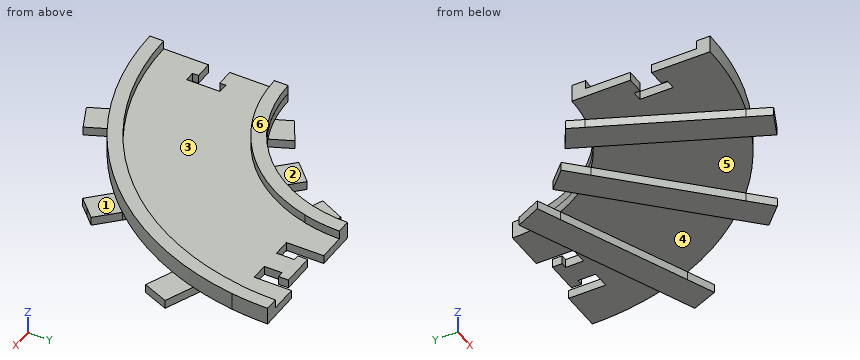
from build123d import *

# Parameters (mm, degrees)
F1_DEPTH  = 3.175
F2_W      = 14.0813224944
F2_H      = 13.6506203337
F3_DEPTH  = 3.175
F5_DEPTH  = 3.175
F2_W_2    = 4.1719265282
F6_DEPTH  = 25.4
F8_DEPTH  = 6.35
F9_DEPTH  = 3.175
F11_DEPTH = 25.4
F13_DEPTH = 3.175


with BuildPart() as f1:
    # F0 (on Top) → F1 (new body)
    with BuildSketch(Plane.XY):
        with BuildLine():
            Line((0, -51.2956328023), (0, -102.09075941))
            ThreePointArc((0, -102.09075941), (72.1890682753, -72.1890682753), (102.09075941, 0))
            Line((102.09075941, 0), (51.2956328023, 0))
            ThreePointArc((51.2956328023, 0), (36.2714897998, -36.2714897998), (0, -51.2956328023))
        make_face()
    extrude(amount=F1_DEPTH)

    # F2 (on Top) → F3 (join)
    with BuildSketch(Plane.XY):
        Polygon((70.5449951161, -7.1183972853), (72.7547951161, -7.1183972853), (72.7547951161, -13.6506203337), (80.5461628969, -13.6506203337), (80.5461628969, -7.1183972853), (82.7559628969, -7.1183972853), (82.7559628969, -3.5022496107), (70.5449951161, -3.5022496107), align=None)
        Polygon((51.7481602728, -13.6506203337), (66.4398123863, -13.6506203337), (66.3695515009, 0), (51.7481602728, 0), align=None)
        with Locations((93.9881238623, -6.8253101669)):
            Rectangle(F2_W, F2_H)
    extrude(amount=F3_DEPTH)

    # F4 (on face) → F5 (join)
    with BuildSketch(Plane.XY.offset(3.175)):
        with BuildLine():
            ThreePointArc((0, -56.3756328023), (39.8635922482, -39.8635922482), (56.3756328023, 0))
            Line((56.3756328023, 0), (51.3330261441, 0))
            ThreePointArc((51.3330261441, 0), (36.2979308853, -36.2979308853), (0, -51.3330261441))
            Line((0, -51.3330261441), (0, -56.3756328023))
        make_face()
        with BuildLine():
            Line((102.09075941, 0), (97.01075941, 0))
            ThreePointArc((97.01075941, 0), (68.5969658269, -68.5969658269), (0, -97.01075941))
            Line((0, -97.01075941), (0, -102.09075941))
            ThreePointArc((0, -102.09075941), (72.1890682753, -72.1890682753), (102.09075941, 0))
        make_face()
    extrude(amount=F5_DEPTH)

    # F2 (on Top) → F6 (cut)
    with BuildSketch(Plane.XY):
        Polygon((51.7481602728, -13.6506203337), (66.4398123863, -13.6506203337), (66.3695515009, 0), (51.7481602728, 0), align=None)
        Polygon((72.7547951161, -13.6506203337), (72.7547951161, -7.1183972853), (70.5449951161, -7.1183972853), (70.5449951161, -3.5022496107), (82.7559628969, -3.5022496107), (82.7559628969, -7.1183972853), (80.5461628969, -7.1183972853), (80.5461628969, -13.6506203337), (86.9474626151, -13.6506203337), (86.9474626151, 0), (76.6565515009, 0), (66.3695515009, 0), (66.4398123863, -13.6506203337), align=None)
        with Locations((93.9881238623, -6.8253101669)):
            Rectangle(F2_W, F2_H)
        with Locations((49.6621970087, -6.8253101669)):
            Rectangle(F2_W_2, F2_H)
    extrude(amount=F6_DEPTH, mode=Mode.SUBTRACT)

    # F7 (on Top) → F8 (join)
    with BuildSketch(Plane.XY):
        with BuildLine():
            ThreePointArc((54.7619331998, -13.660392724), (56.0189261095, -6.8815386855), (56.4400182242, 0))
            Line((56.4400182242, 0), (51.3051767249, 0))
            ThreePointArc((51.3051767249, 0), (50.8400637591, -6.8926827684), (49.4531579316, -13.660392724))
            Line((49.4531579316, -13.660392724), (54.7619331998, -13.660392724))
        make_face()
        with BuildLine():
            Line((102.1051767249, 0), (97.1390098326, 0))
            ThreePointArc((97.1390098326, 0), (96.8973822865, -6.8472284381), (96.1737017167, -13.660392724))
            Line((96.1737017167, -13.660392724), (101.1872560388, -13.660392724))
            ThreePointArc((101.1872560388, -13.660392724), (101.8754380952, -6.8455990928), (102.1051767249, 0))
        make_face()
    extrude(amount=F8_DEPTH)

    # F2 (on Top) → F9 (join)
    with BuildSketch(Plane.XY):
        with Locations((93.9881238623, -6.8253101669)):
            Rectangle(F2_W, F2_H)
        Polygon((51.7481602728, -13.6506203337), (66.4398123863, -13.6506203337), (66.3695515009, 0), (51.7481602728, 0), align=None)
    extrude(amount=F9_DEPTH)

    # F10 (on face) → F11 (cut)
    with BuildSketch(Plane.XY.offset(3.175)):
        Polygon((6.3110076786, -72.776100911), (0, -72.776100911), (0, -80.5674686917), (6.3110076786, -80.5674686917), (6.3110076786, -82.7772686917), (10.0084030033, -82.7772686917), (10.0084030033, -70.566300911), (6.3110076786, -70.566300911), align=None)
    extrude(amount=-F11_DEPTH, mode=Mode.SUBTRACT)

    # F12 (on face) → F13 (join)
    with BuildSketch(Plane(origin=(0, 0, 0), x_dir=(1, 0, 0), z_dir=(0, 0, -1))):
        with BuildLine():
            ThreePointArc((39.6434592285, 32.5520826521), (37.980845771, 34.4774897449), (36.2248193412, 36.3181002847))
            Line((36.2248193412, 36.3181002847), (29.0498583475, 29.1246633635))
            Line((29.0498583475, 29.1246633635), (32.646576808, 25.5371828667))
            Line((32.646576808, 25.5371828667), (39.6434592285, 32.5520826521))
        make_face()
        with BuildLine():
            Line((29.0498583475, 29.1246633635), (36.2248193412, 36.3181002847))
            ThreePointArc((36.2248193412, 36.3181002847), (34.3796988436, 38.0693873344), (32.4500223073, 39.7270436459))
            Line((32.4500223073, 39.7270436459), (25.4531398869, 32.7121438604))
            Line((25.4531398869, 32.7121438604), (29.0498583475, 29.1246633635))
        make_face()
        with BuildLine():
            Line((36.2248193412, 36.3181002847), (72.0961827352, 72.2818344532))
            ThreePointArc((72.0961827352, 72.2818344532), (70.2749350461, 74.0537417095), (68.4101530773, 75.7797737714))
            Line((68.4101530773, 75.7797737714), (32.4500223073, 39.7270436459))
            ThreePointArc((32.4500223073, 39.7270436459), (34.3796988436, 38.0693873344), (36.2248193412, 36.3181002847))
        make_face()
        with BuildLine():
            ThreePointArc((75.6035899985, 68.6048127777), (73.8727679087, 70.4651496728), (72.0961827352, 72.2818344532))
            Line((72.0961827352, 72.2818344532), (36.2248193412, 36.3181002847))
            ThreePointArc((36.2248193412, 36.3181002847), (37.980845771, 34.4774897449), (39.6434592285, 32.5520826521))
            Line((39.6434592285, 32.5520826521), (75.6035899985, 68.6048127777))
        make_face()
        with BuildLine():
            Line((79.271143729, 79.4752713743), (72.0961827352, 72.2818344532))
            ThreePointArc((72.0961827352, 72.2818344532), (73.8727679087, 70.4651496728), (75.6035899985, 68.6048127777))
            Line((75.6035899985, 68.6048127777), (82.8785053866, 75.8984614814))
            Line((82.8785053866, 75.8984614814), (79.271143729, 79.4752713743))
        make_face()
        with BuildLine():
            ThreePointArc((68.4101530773, 75.7797737714), (70.2749350461, 74.0537417095), (72.0961827352, 72.2818344532))
            Line((72.0961827352, 72.2818344532), (79.271143729, 79.4752713743))
            Line((79.271143729, 79.4752713743), (75.7328631666, 83.1213402502))
            Line((75.7328631666, 83.1213402502), (68.4101530773, 75.7797737714))
        make_face()
        with BuildLine():
            Line((20.0341812257, 47.2215366883), (40.6881574418, 93.6322433828))
            ThreePointArc((40.6881574418, 93.6322433828), (35.9596571955, 95.5480309127), (31.1413521737, 97.2251991086))
            Line((31.1413521737, 97.2251991086), (10.2418471319, 50.2627746142))
            ThreePointArc((10.2418471319, 50.2627746142), (15.2141958482, 48.9874493037), (20.0341812257, 47.2215366883))
        make_face()
        with BuildLine():
            ThreePointArc((31.1413521737, 97.2251991086), (35.9596571955, 95.5480309127), (40.6881574418, 93.6322433828))
            Line((40.6881574418, 93.6322433828), (44.0618023276, 101.2130230665))
            Line((44.0618023276, 101.2130230665), (34.7585338749, 105.353220427))
            Line((34.7585338749, 105.353220427), (31.1413521737, 97.2251991086))
        make_face()
        with BuildLine():
            Line((16.5176168084, 39.3196083605), (20.0341812257, 47.2215366883))
            ThreePointArc((20.0341812257, 47.2215366883), (15.2141958482, 48.9874493037), (10.2418471319, 50.2627746142))
            Line((10.2418471319, 50.2627746142), (7.7137911807, 44.5820833017))
            Line((7.7137911807, 44.5820833017), (16.5176168084, 39.3196083605))
        make_face()
        with BuildLine():
            ThreePointArc((49.4459554372, 13.6506203337), (48.462460254, 16.8116593685), (47.2771132537, 19.902675875))
            Line((47.2771132537, 19.902675875), (38.7149937451, 16.3121093065))
            Line((38.7149937451, 16.3121093065), (43.1567628434, 7.0787111473))
            Line((43.1567628434, 7.0787111473), (50.3058721439, 10.0767249947))
            ThreePointArc((50.3058721439, 10.0767249947), (49.9128620494, 11.8712830314), (49.4558563093, 13.6506203337))
            Line((49.4558563093, 13.6506203337), (49.4459554372, 13.6506203337))
        make_face()
        with BuildLine():
            ThreePointArc((97.6098508897, 29.9138791566), (95.9858944102, 34.7740022313), (94.1201154327, 39.5465172658))
            Line((94.1201154327, 39.5465172658), (47.2771132537, 19.902675875))
            ThreePointArc((47.2771132537, 19.902675875), (48.462460254, 16.8116593685), (49.4459554372, 13.6506203337))
            Line((49.4459554372, 13.6506203337), (49.4558563093, 13.6506203337))
            ThreePointArc((49.4558563093, 13.6506203337), (49.9128620494, 11.8712830314), (50.3058721439, 10.0767249947))
            Line((50.3058721439, 10.0767249947), (97.6098508897, 29.9138791566))
        make_face()
        with BuildLine():
            Line((104.0109246969, 43.6942763627), (94.1201154327, 39.5465172658))
            ThreePointArc((94.1201154327, 39.5465172658), (95.9858944102, 34.7740022313), (97.6098508897, 29.9138791566))
            Line((97.6098508897, 29.9138791566), (107.9681979582, 34.2577025116))
            Line((107.9681979582, 34.2577025116), (104.0109246969, 43.6942763627))
        make_face()
    extrude(amount=F13_DEPTH)


solid = f1.part
Source: CAD feature listing. Evaluate the final solid. Frame: model axes, mm. Face numbers are marked on the shaded views. A direction names the side the tool comes from. Coordinates: 2 decimals unless noted, no trailing zeros. Write each loop counter-clockwise with the first axis right and the second up, starting at its lowest first coordinate (ties: lowest second). Pieces come first, ordered by that corner, then holes. Notation, with made-up numbers: M 53,86 L 65,86 A18 cw 65,107 Z; hole C 5,28 d4. An arc over 180 degrees is marked long. Use a Markdown table: item, result.
1) Reachability of the marked faces 1, 2, 3 and 4 from +Z, -Z, +X, -X, +Y, -Y: full face, straight path, thin tool, end or side. Return the list, or none.
Conclusion:
| item | result |
|---|---|
| face 1 | +Z, +X, -Y |
| face 2 | +Z, -X, +Y |
| face 3 | +Z |
| face 4 | -Z |
2) First-contact query: pin 1 Ø2.5 at (y, z) = (-72, 1.5) entering from +X; pin 2 Ø3.5 at (x, z) = (2.5, 1.5) entering from +Y; pin 3 Ø4 at (x, z) = (35.5, 1) entering from +Y; pin 4 Ø10 at (x, y) = (31, -19.5) entering from -Z. Flat tips, straight axial feed; report the tip coordinate or a pass-through.
Conclusion:
| item | result |
|---|---|
| pin 1 | stops at x = 73.6 |
| pin 2 | stops at y = -51.12 |
| pin 3 | stops at y = -26.66 |
| pin 4 | passes through |
3) Ray query, L1, parallel to Z at x = 37, y = -57.5 (3 decimals); L2, parallel to Z at x = 29, y = -85 (3 decimals); L3, parallel to Y at x = 26, z = -2. Return the intervals inside material, ascending.
Conclusion:
| item | result |
|---|---|
| L1 | z = 0 to 3.175 |
| L2 | z = -3.175 to 3.175 |
| L3 | y = -85.67 to -60.63, -33.26 to -32.17 |
4) Mould query, pull axis X, two halves, no side actions, for the marked faces 5 and 6. Classes: pulls with the +X half, pulls with the -X half, needs draft (parallel to the pull), parting line crosses it, or undercut.
Conclusion:
| item | result |
|---|---|
| face 5 | undercut |
| face 6 | needs draft |
5) Section B-B, the plane z = -1.5. Output: boundary loops of the cut face in (x, y) (1 decimal), then the cut area to 3 significant figures.
Conclusion:
| item | result |
|---|---|
| outline | M 7.7,-44.6 L 34.8,-105.4 L 44.1,-101.2 L 16.5,-39.3 Z; M 25.5,-32.7 L 75.7,-83.1 L 79.3,-79.5 L 82.9,-75.9 L 32.6,-25.5 Z; M 38.7,-16.3 L 104,-43.7 L 108,-34.3 L 43.2,-7.1 Z |
| area | 2,130 mm^2 |
6) Section D-D, the plane y = -89.5. Output: boundary loops of the cut face in (x, z) (3 decimals).
Conclusion:
| item | result |
|---|---|
| outline | M 0,0 L 27.703,0 L 27.703,-3.175 L 38.849,-3.175 L 38.849,0 L 49.115,0 L 49.115,6.35 L 37.428,6.35 L 37.428,3.175 L 0,3.175 Z |
7) Section C-C, the plane x = 27. Output: boundary loops of the cut face in (y, z) (3 decimals).
Conclusion:
| item | result |
|---|---|
| outline | M -98.456,0 L -87.919,0 L -87.919,-3.175 L -62.874,-3.175 L -62.874,0 L -43.615,0 L -43.615,3.175 L -43.659,3.175 L -43.659,6.35 L -49.49,6.35 L -49.49,3.175 L -93.178,3.175 L -93.178,6.35 L -98.456,6.35 Z; M -34.263,-3.175 L -31.169,-3.175 L -31.169,0 L -34.263,0 Z |
